```python
from build123d import *

# Parameters (mm, degrees)
SALIENTE_EXTRUIR1_DEPTH = 6
CROQUIS4_R              = 2
CORTAR_EXTRUIR1_DEPTH   = 15


with BuildPart() as part:
    # Croquis1 → Saliente-Extruir1 (new body)
    with BuildSketch(Plane.XY):
        with BuildLine():
            Line((7.5, -36.38301994), (2.5, -36.38301994))
            Line((2.5, -36.38301994), (2.5, -26.38301994))
            Line((2.5, -26.38301994), (-2.5, -26.38301994))
            Line((-2.5, -26.38301994), (-2.5, -36.38301994))
            Line((-2.5, -36.38301994), (-7.5, -36.38301994))
            Line((-7.5, -36.38301994), (-7.5, -26.38301994))
            Line((-7.5, -26.38301994), (-7.101695438, -26.38301994))
            Line((-7.101695438, -26.38301994), (-5, 0))
            ThreePointArc((-5, 0), (0, 5), (5, 0))
            Line((5, 0), (7.101695438, -26.38301994))
            Line((7.101695438, -26.38301994), (7.5, -26.38301994))
            Line((7.5, -26.38301994), (7.5, -36.38301994))
        make_face()
    extrude(amount=SALIENTE_EXTRUIR1_DEPTH)

    # Croquis2 → Cortar-Revolución1 (revolve, cut)
    with BuildSketch(Plane(origin=(0, 0, 0), x_dir=(0, 0, -1), z_dir=(1, 0, 0))):
        with BuildLine():
            Line((3, 0), (-5, 0))
            ThreePointArc((-5, 0), (-1, 4), (3, 0))
        make_face()
    revolve(axis=Axis((0, 0, -3), (0, 0, 1)), mode=Mode.SUBTRACT)

    # Croquis4 → Cortar-Extruir1 (cut)
    with BuildSketch(Plane(origin=(7.5, 0, 0), x_dir=(0, 0, -1), z_dir=(1, 0, 0))):
        with Locations((-3, -31.38301994)):
            Circle(CROQUIS4_R)
    extrude(amount=-CORTAR_EXTRUIR1_DEPTH, mode=Mode.SUBTRACT)

    # Croquis5 → Cortar-Revolución2 (revolve, cut)
    with BuildSketch(Plane(origin=(0, 0, 0), x_dir=(0, 0, -1), z_dir=(1, 0, 0))):
        with BuildLine():
            Line((-7, -31.38301994), (1, -31.38301994))
            ThreePointArc((1, -31.38301994), (-3, -27.38301994), (-7, -31.38301994))
        make_face()
    revolve(axis=Axis((0, -31.38301994, 7), (0, 0, -1)), mode=Mode.SUBTRACT)


solid = part.part
```
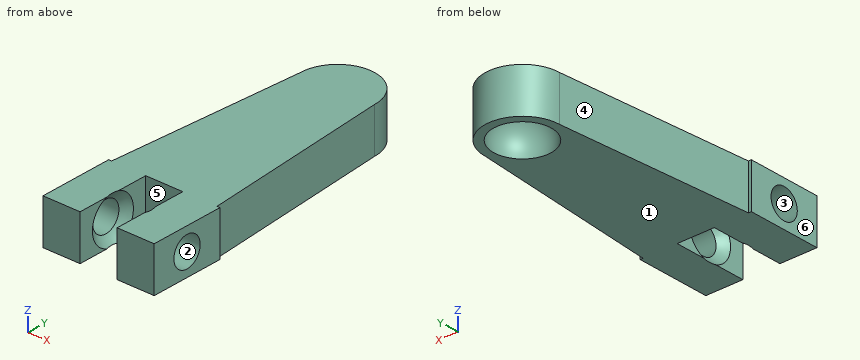
Build history of the part. All positions in model axes, mm. Face numbers are marked on the shaded views. A direction names the side the tool comes from. Round coordinates to 2 decimals unless told otherwise and drop trailing zeros. Loops run counter-clockwise (first coordinate to the right, second up) from the corner with the lowest first, then second, coordinate; pieces in that order, holes last. Notation, with made-up numbers: M 5,-16 L 48,-16 A7 ccw 48,-5 Z; hole C 27.5,13.5 d8. An arc over 180 degrees is marked long. Answer as CSV lines item,"result".
1. Cut at D-D on x = 0. Write the cut outline in (y, z).
Resolved:
outline,"M -26.38,0 L -3.87,0 A4 cw long 3.87,0 L 5,0 L 5,6 L -26.38,6 Z"
2. 3-axis set-ups, long thin cutter, end or side, ignore diameter. For the marked faces 5 and 6: which of +Z, -Z, +X, -X, +Y, -Y reach the whole face in a straight line?
Resolved:
face 5,"+Z, -Z, -Y"
face 6,"+Z, -Z, -X, +Y, -Y"
3. Two-plate mould, pull along Z, no slides. Class the marked faces 1, 2, 3 and 4: released by +Z, released by -Z, zero draft, split by the parting line, or undercut.
Resolved:
face 1,"released by -Z"
face 2,"undercut"
face 3,"undercut"
face 4,"zero draft"
4. Cut at B-B on x = -6.25. Write the cut outline in (y, z).
Resolved:
outline,"M -36.38,0 L -15.69,0 L -15.69,6 L -36.38,6 Z; hole C -31.38,3 d4"
5. Flat gauge pins, fed straight in: P1, Ø2, axis at x = 1, z = 3.5, coming from the -Y side; P2, Ø1, axis at y = -25, z = 5.5, coming from the +X side. Where does each tip first touch, or does it go through?
Resolved:
P1,"stops at y = -26.38"
P2,"stops at x = 7.03"
6. Cut at C-C on y = -6.5. Write the cut outline in (x, z).
Resolved:
outline,"M -5.52,0 L 5.52,0 L 5.52,6 L -5.52,6 Z"
7. Wall check: probe 1 along X at (y, z) = (-28.5, 1); probe 2 along Y at (x, z) = (1.25, 1.75); probe 3 along X at (y, z) = (3, 1.25). Give the ranges that are in metal, low to high. Write a range as [from, to].
Resolved:
probe 1,"x = [-7.5, -2.5], [2.5, 7.5]"
probe 2,"y = [-26.38, -3.72], [3.72, 4.84]"
probe 3,"x = [-4, -2.63], [2.63, 4]"
8. Cut at A-A on z = 3. Write the cut outline in (x, y), then the cut area to 3 significant figures.
Resolved:
outline,"M -7.5,-36.38 L -2.5,-36.38 L -2.5,-34.51 A4 cw -3.46,-33.38 L -7.5,-33.38 Z; M -7.5,-29.38 L -3.46,-29.38 A4 cw -2.5,-28.26 L -2.5,-26.38 L 2.5,-26.38 L 2.5,-28.26 A4 cw 3.46,-29.38 L 7.5,-29.38 L 7.5,-26.38 L 7.1,-26.38 L 5,0 A5 ccw -5,0 L -7.1,-26.38 L -7.5,-26.38 Z; M 2.5,-36.38 L 7.5,-36.38 L 7.5,-33.38 L 3.46,-33.38 A4 cw 2.5,-34.51 Z; hole C 0,0 d6.93"
area,"378 mm²"
